Work out the finished part from the listing and answer in its coordinate system (mm). Face numbers are marked on the shaded views. A direction names the side the tool comes from. Round coordinates to 2 decimals unless told otherwise and drop trailing zeros. Loops run counter-clockwise (first coordinate to the right, second up) from the corner with the lowest first, then second, coordinate; pieces in that order, holes last. Notation, with made-up numbers: (-22, 69) -> (22, 69) arc R25 ccw to (22, 91) -> close; hole circle Ø1 at (-10.5, 2). An arc over 180 degrees is marked (long way). Use one line per item in the form item = value.
```python
from build123d import *

# Parameters (mm, degrees)
F0_R     = 20
F1_DEPTH = 25
F2_R     = 11.05
F3_DEPTH = 15
F4_R     = 11.05
F4_R_2   = 7.5
F5_DEPTH = 8


with BuildPart() as f1:
    # F0 (on Top) → F1 (new body)
    with BuildSketch(Plane.XY):
        Circle(F0_R)
    extrude(amount=F1_DEPTH)

    # F2 (on face) → F3 (cut)
    with BuildSketch(Plane.XY.offset(25)):
        Circle(F2_R)
    extrude(amount=-F3_DEPTH, mode=Mode.SUBTRACT)

    # F4 (on face) → F5 (join)
    with BuildSketch(Plane.XY.offset(10)):
        Circle(F4_R)
        Circle(F4_R_2, mode=Mode.SUBTRACT)
    extrude(amount=F5_DEPTH)


solid = f1.part
```
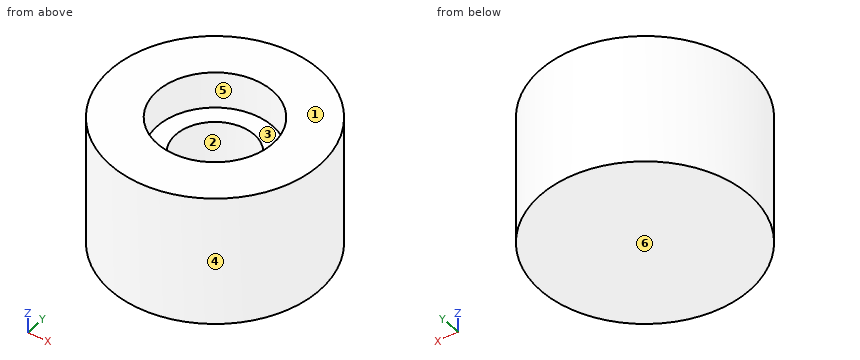
(1) Find section C-C, the plane z = 4.25. Write down the section's boundary in (x, y), then the cut area to 3 significant figures.
Completed:
outline = circle Ø40 at (0, 0)
area = 1,260 mm2
(2) Find section D-D, the plane z = 21. Write down the section's boundary in (x, y).
Completed:
outline = circle Ø40 at (0, 0); hole circle Ø22.1 at (0, 0)
(3) Given P1, Ø4.5, axis at x = -3, y = -0.5, coming from the +Z side; P2, Ø17, axis at x = 0, y = 0, coming from the -Z side; P3, Ø3, axis at y = 13, z = 11, coming from the -X side; P4, Ø1.5, axis at y = -3, z = 4, coming from the +X side, each flat-ended and moving along its own axis, determine where each tip first touches the part or whether it passes through.
Completed:
P1 = 10
P2 = 0
P3 = -16.36
P4 = 19.87
(4) Consider L1, parallel to Y at x = 0, z = 15.25; L2, parallel to Y at x = 0, z = 19.75; L3, parallel to Z at x = -8.5, y = -1. Determine where each line is inside the solid, lowest interval first.
Completed:
L1 = -20 to -7.5, 7.5 to 20
L2 = -20 to -11.05, 11.05 to 20
L3 = 0 to 18
(5) Find section A-A, the plane x = 0. Write down the section's boundary in (y, z), then the cut area to 3 significant figures.
Completed:
outline = (-20, 0) -> (20, 0) -> (20, 25) -> (11.05, 25) -> (11.05, 18) -> (7.5, 18) -> (7.5, 10) -> (-7.5, 10) -> (-7.5, 18) -> (-11.05, 18) -> (-11.05, 25) -> (-20, 25) -> close
area = 725 mm2
(6) For a pull along X with two mould halves and no side action, classify the marked faces 1, 2, 3 and 4 as +X half, -X half, draft (parallel to the pull), parting line (faces both ways), or undercut.
Completed:
face_1 = draft
face_2 = undercut
face_3 = undercut
face_4 = parting line
(7) For the marked faces 5 and 6, determine the directions among +Z, -Z, +X, -X, +Y, -Y from which every point of the face is accessible in a straight line to the end or side of a thin tool.
Completed:
face_5 = +Z
face_6 = -Z, +X, -X, +Y, -Y
